from build123d import *

# Parameters (mm, degrees)
F0_W     = 139
F0_H     = 40
F0_W_2   = 10
F0_H_2   = 10
F1_DEPTH = 2
F2_SIZE  = 1


with BuildPart() as f1:
    # F0 (on Top) → F1 (new body)
    with BuildSketch(Plane.XY):
        with Locations((60.5, 11)):
            Rectangle(F0_W, F0_H)
        Rectangle(F0_W_2, F0_H_2, mode=Mode.SUBTRACT)
        with Locations((11, 0)):
            Rectangle(F0_W_2, F0_H_2, mode=Mode.SUBTRACT)
        with Locations((22, 0)):
            Rectangle(F0_W_2, F0_H_2, mode=Mode.SUBTRACT)
        with Locations((33, 0)):
            Rectangle(F0_W_2, F0_H_2, mode=Mode.SUBTRACT)
        with Locations((44, 0)):
            Rectangle(F0_W_2, F0_H_2, mode=Mode.SUBTRACT)
        with Locations((55, 0)):
            Rectangle(F0_W_2, F0_H_2, mode=Mode.SUBTRACT)
        with Locations((66, 0)):
            Rectangle(F0_W_2, F0_H_2, mode=Mode.SUBTRACT)
        with Locations((77, 0)):
            Rectangle(F0_W_2, F0_H_2, mode=Mode.SUBTRACT)
        with Locations((88, 0)):
            Rectangle(F0_W_2, F0_H_2, mode=Mode.SUBTRACT)
        with Locations((99, 0)):
            Rectangle(F0_W_2, F0_H_2, mode=Mode.SUBTRACT)
        with Locations((110, 0)):
            Rectangle(F0_W_2, F0_H_2, mode=Mode.SUBTRACT)
        with Locations((121, 0)):
            Rectangle(F0_W_2, F0_H_2, mode=Mode.SUBTRACT)
        with Locations((0, 11)):
            Rectangle(F0_W_2, F0_H_2, mode=Mode.SUBTRACT)
        with Locations((11, 11)):
            Rectangle(F0_W_2, F0_H_2, mode=Mode.SUBTRACT)
        with Locations((22, 11)):
            Rectangle(F0_W_2, F0_H_2, mode=Mode.SUBTRACT)
        with Locations((33, 11)):
            Rectangle(F0_W_2, F0_H_2, mode=Mode.SUBTRACT)
        with Locations((44, 11)):
            Rectangle(F0_W_2, F0_H_2, mode=Mode.SUBTRACT)
        with Locations((55, 11)):
            Rectangle(F0_W_2, F0_H_2, mode=Mode.SUBTRACT)
        with Locations((0, 22)):
            Rectangle(F0_W_2, F0_H_2, mode=Mode.SUBTRACT)
        with Locations((11, 22)):
            Rectangle(F0_W_2, F0_H_2, mode=Mode.SUBTRACT)
        with Locations((22, 22)):
            Rectangle(F0_W_2, F0_H_2, mode=Mode.SUBTRACT)
        with Locations((33, 22)):
            Rectangle(F0_W_2, F0_H_2, mode=Mode.SUBTRACT)
        with Locations((44, 22)):
            Rectangle(F0_W_2, F0_H_2, mode=Mode.SUBTRACT)
        with Locations((55, 22)):
            Rectangle(F0_W_2, F0_H_2, mode=Mode.SUBTRACT)
        with Locations((66, 11)):
            Rectangle(F0_W_2, F0_H_2, mode=Mode.SUBTRACT)
        with Locations((77, 11)):
            Rectangle(F0_W_2, F0_H_2, mode=Mode.SUBTRACT)
        with Locations((88, 11)):
            Rectangle(F0_W_2, F0_H_2, mode=Mode.SUBTRACT)
        with Locations((99, 11)):
            Rectangle(F0_W_2, F0_H_2, mode=Mode.SUBTRACT)
        with Locations((110, 11)):
            Rectangle(F0_W_2, F0_H_2, mode=Mode.SUBTRACT)
        with Locations((121, 11)):
            Rectangle(F0_W_2, F0_H_2, mode=Mode.SUBTRACT)
        with Locations((66, 22)):
            Rectangle(F0_W_2, F0_H_2, mode=Mode.SUBTRACT)
        with Locations((77, 22)):
            Rectangle(F0_W_2, F0_H_2, mode=Mode.SUBTRACT)
        with Locations((88, 22)):
            Rectangle(F0_W_2, F0_H_2, mode=Mode.SUBTRACT)
        with Locations((99, 22)):
            Rectangle(F0_W_2, F0_H_2, mode=Mode.SUBTRACT)
        with Locations((110, 22)):
            Rectangle(F0_W_2, F0_H_2, mode=Mode.SUBTRACT)
        with Locations((121, 22)):
            Rectangle(F0_W_2, F0_H_2, mode=Mode.SUBTRACT)
    extrude(amount=F1_DEPTH)

    # F2
    f2_edges = [f1.edges().sort_by_distance(p)[0] for p in [
        (60.5, -9, 2),
        (-9, 11, 2),
        (60.5, 31, 2),
        (130, 11, 2),
    ]]
    chamfer(f2_edges, length=F2_SIZE)


solid = f1.part
Input: part model. Units: mm. Frame: model coordinates. Give positions to 0.01 mm unless a question says otherwise; leave off trailing zeros. Order: outer loops, then holes, each group sorted by start corner. A loop starts at its lowest first (then second) coordinate and runs counter-clockwise, first axis right, second up. Notation, with made-up numbers: (41, 12.25) - (96, 12.25) arc R32 ccw to (96, 45.25) - close; hole circle Ø10 at (-32, -25.5). An arc over 180 degrees is marked (long way). Answer as a JSON object with one key per item and string values. Group by question number.
Q1. Line query: probe 1 along Y at (x, z) = (118.5, 0.7); probe 2 along Y at (x, z) = (68, 1.1); probe 3 along Y at (x, z) = (27.5, 1.55). Output: solid intervals per line, ascending.
Q2. Cut plane A-A, the plane x = 65. Output: boundary loops of the cut face in (y, z), then the cut area to 3 significant figures.
Q3. Cut plane B-B, the plane y = 1. Count the separate pieces of the cut face and the enclosed holes in it, then the cut area to 3 significant figures.
Results:
{
 "1": {"probe 1": "-9 to -5, 5 to 6, 16 to 17, 27 to 31", "probe 2": "-8.9 to -5, 5 to 6, 16 to 17, 27 to 30.9", "probe 3": "-8.45 to 30.45"},
 "2": {"outline": "(-9, 0) - (-5, 0) - (-5, 2) - (-8, 2) - (-9, 1) - close; (5, 0) - (6, 0) - (6, 2) - (5, 2) - close; (16, 0) - (17, 0) - (17, 2) - (16, 2) - close; (27, 0) - (31, 0) - (31, 1) - (30, 2) - (27, 2) - close", "area": "19.0 mm^2"},
 "3": {"separate pieces": "13", "enclosed holes": "0", "area": "37.0 mm^2"}
}
